from build123d import *

# Parameters (mm, degrees)
BOSS_EXTRUDE1_DEPTH = 3.5
SKETCH2_R           = 3.3
BOSS_EXTRUDE2_DEPTH = 0.5
SKETCH3_W           = 3
SKETCH3_H           = 3
BOSS_EXTRUDE3_DEPTH = 2.8
SKETCH4_R           = 6.5
BOSS_EXTRUDE4_DEPTH = 1
SKETCH5_R           = 5.75
BOSS_EXTRUDE5_DEPTH = 4.5
FILLET1_R           = 0.2


with BuildPart() as part:
    # Sketch1 → Boss-Extrude1 (new body)
    with BuildSketch(Plane(origin=(0, 0, 0), x_dir=(1, 0, 0), z_dir=(0, 1, 0))):
        with BuildLine():
            Line((-0.5, 0), (-11.5, 0))
            ThreePointArc((-11.5, 0), (-11.853553391, 0.146446609), (-12, 0.5))
            Line((-12, 0.5), (-12, 11.5))
            ThreePointArc((-12, 11.5), (-11.853553391, 11.853553391), (-11.5, 12))
            Line((-11.5, 12), (-0.5, 12))
            ThreePointArc((-0.5, 12), (-0.146446609, 11.853553391), (0, 11.5))
            Line((0, 11.5), (0, 0.5))
            ThreePointArc((0, 0.5), (-0.146446609, 0.146446609), (-0.5, 0))
        make_face()
    extrude(amount=BOSS_EXTRUDE1_DEPTH)

    # Sketch2 → Boss-Extrude2 (add)
    with BuildSketch(Plane(origin=(0, 3.5, 0), x_dir=(1, 0, 0), z_dir=(0, 1, 0))):
        with Locations(Location((-6, 6, 0), (0, 0, 270))):
            Circle(SKETCH2_R)
    extrude(amount=BOSS_EXTRUDE2_DEPTH)

    # Sketch3 → Boss-Extrude3 (add)
    with BuildSketch(Plane(origin=(0, 4, 0), x_dir=(1, 0, 0), z_dir=(0, 1, 0))):
        with Locations((-6, 6)):
            Rectangle(SKETCH3_W, SKETCH3_H)
    extrude(amount=BOSS_EXTRUDE3_DEPTH)

    # Sketch4 → Boss-Extrude4 (add)
    with BuildSketch(Plane(origin=(0, 6.8, 0), x_dir=(1, 0, 0), z_dir=(0, 1, 0))):
        with Locations(Location((-6, 6, 0), (0, 0, 270))):
            Circle(SKETCH4_R)
    extrude(amount=BOSS_EXTRUDE4_DEPTH)

    # Sketch5 → Boss-Extrude5 (add)
    with BuildSketch(Plane(origin=(0, 7.8, 0), x_dir=(1, 0, 0), z_dir=(0, 1, 0))):
        with Locations(Location((-6, 6, 0), (0, 0, 270))):
            Circle(SKETCH5_R)
    extrude(amount=BOSS_EXTRUDE5_DEPTH)

    # Fillet1
    fillet1_edges = [part.edges().sort_by_distance(p)[0] for p in [
        (-6, 7.8, -12.5),
        (-6, 12.3, -11.75),
    ]]
    fillet(fillet1_edges, radius=FILLET1_R)


solid = part.part
Work out the finished part from the listing and answer in its coordinate system (mm). A direction names the side the tool comes from. Give positions to 0.01 mm unless a question says otherwise; leave off trailing zeros. Write each loop counter-clockwise with the first axis right and the second up, starting at its lowest first coordinate (ties: lowest second). Pieces come first, ordered by that corner, then holes. Notation, with made-up numbers: (21.5, 21) - (75.5, 21) arc R11 cw to (75.5, 34) - close; hole circle Ø5 at (63, -27). An arc over 180 degrees is marked (long way). One line per item, written item: value. Start each with the question number.
1. Find section A-A (y = 1.5). Write down the section's boundary in (x, z), then the cut area to 3 significant figures.
2. Find section C-C (z = -6). Write down the section's boundary in (x, y), then the cut area to 3 significant figures.
3. For a pull along Y with two mould halves and no side action, classify faces 1 (the flat face through (-6, 0, -6)), 2 (the flat face through (-6, 5, -7.5)), 3 (the flat face through (-6, 12.3, -6)), 4 (the flat face through (-12, 2, -6)) as +Y half, -Y half, draft (parallel to the pull), parting line (faces both ways), or undercut.
4. Find section D-D (y = 7.25). Write down the section's boundary in (x, z), then the cut area to 3 significant figures.
5. Given pin 1 (5 mm diameter, centred on x = -10.5, y = 3, fed in from +Z); pin 2 (3 mm diameter, centred on y = 1, z = -5.5, fed in from +X); pin 3 (3 mm diameter, centred on x = -6.5, y = 5.5, fed in from -Z); pin 4 (1 mm diameter, centred on x = -5.5, y = 1, fed in from -Z), each flat-ended and moving along its own axis, determine where each tip first touches the part or whether it passes through.
6. Find section B-B (x = -6). Write down the section's boundary in (y, z).
7. Consider probe 1 along Y at (x, z) = (-4, -6.25); probe 2 along Y at (x, z) = (-1.5, -9.25); probe 3 along Z at (x, y) = (-5.75, 2.5). Determine where each line is inside the solid, lowest interval first.
8. For faces 5 (the cylindrical face through (-0.3, 9.92, -6.75)), 6 (the cylindrical face through (-7.26, 3.75, -2.95)), 7 (the flat face through (-6, 5, -4.5)), 8 (the flat face through (-6, 2, 0)), 9 (the flat face through (-4.5, 5, -6)), determine the directions among +Z, -Z, +X, -X, +Y, -Y from which every point of the face is accessible in a straight line to the end or side of a thin tool.
Geometry results:
1. outline: (-12, -11.5) arc R0.5 ccw to (-11.5, -12) - (-0.5, -12) arc R0.5 ccw to (0, -11.5) - (0, -0.5) arc R0.5 ccw to (-0.5, 0) - (-11.5, 0) arc R0.5 ccw to (-12, -0.5) - close
1. area: 144 mm2
2. outline: (-12.5, 6.8) - (-7.5, 6.8) - (-7.5, 4) - (-9.3, 4) - (-9.3, 3.5) - (-12, 3.5) - (-12, 0) - (0, 0) - (0, 3.5) - (-2.7, 3.5) - (-2.7, 4) - (-4.5, 4) - (-4.5, 6.8) - (0.5, 6.8) - (0.5, 7.6) arc R0.2 ccw to (0.3, 7.8) - (-0.25, 7.8) - (-0.25, 12.1) arc R0.2 ccw to (-0.45, 12.3) - (-11.55, 12.3) arc R0.2 ccw to (-11.75, 12.1) - (-11.75, 7.8) - (-12.3, 7.8) arc R0.2 ccw to (-12.5, 7.6) - close
2. area: 118 mm2
3. face 1: -Y half
3. face 2: undercut
3. face 3: +Y half
3. face 4: draft
4. outline: circle Ø13 at (-6, -6)
4. area: 133 mm2
5. pin 1: z = 0
5. pin 2: x = 0
5. pin 3: z = -12.5
5. pin 4: z = -12
6. outline: (0, -12) - (3.5, -12) - (3.5, -9.3) - (4, -9.3) - (4, -7.5) - (6.8, -7.5) - (6.8, -12.5) - (7.6, -12.5) arc R0.2 ccw to (7.8, -12.3) - (7.8, -11.75) - (12.1, -11.75) arc R0.2 ccw to (12.3, -11.55) - (12.3, -0.45) arc R0.2 ccw to (12.1, -0.25) - (7.8, -0.25) - (7.8, 0.3) arc R0.2 ccw to (7.6, 0.5) - (6.8, 0.5) - (6.8, -4.5) - (4, -4.5) - (4, -2.7) - (3.5, -2.7) - (3.5, 0) - (0, 0) - close
7. probe 1: 0 to 4, 6.8 to 12.3
7. probe 2: 0 to 3.5, 6.8 to 12.3
7. probe 3: -12 to 0
8. face 5: +Y
8. face 6: none
8. face 7: +Z, +X, -X
8. face 8: +Z, +X, -X, -Y
8. face 9: +Z, -Z, +X
